Here's the drawing with two shaded views (mm, measured from the low corner). I have some questions. A direction names the side the tool comes from. Give positions to 0.01 mm unless a question says otherwise; leave off trailing zeros. Loops run counter-clockwise (first coordinate to the right, second up) from the corner with the lowest first, then second, coordinate; pieces in that order, holes last. Notation, with made-up numbers: M 32,77 L 48,77 A26 cw 48,91 Z; hole C 56.5,85.5 d9. An arc over 180 degrees is marked long. Put each result on its own line as item: value. Start each with the question number.
1) Imagine slicing it at B-B (z = 5.5). State how many separate pieces and enclosed holes the cut face has, then the cut area to 3 significant figures.
2) For the marked faces 4 and 5, which set-ups out of +Z, -Z, +X, -X, +Y, -Y let a thin tool reach every point of the face, with its end or its side?
3) Imagine slicing it at A-A (y = 5). Write out the boundary of the cut face in (x, z) (1 decimal).
4) If we mould it in two halves opening along X, with no side actions, what happens to the marked faces 1, 2 and 3? For each: +X half, -X half, draft (parallel to the pull), parting line (faces both ways), or undercut.
5) Please list where these lines run through material, in increasing order: line 1 along X through (y, z) = (1.5, 2.5); line 2 along X through (y, z) = (2.75, 5.25); line 3 along X through (y, z) = (4.5, 7) (1 decimal). Write a range as from..to.
6) For P1, Ø1.6, axis at y = 2, z = 3, coming from the -X side; P2, Ø1, axis at x = 41, z = 3.5, coming from the +Y side (1 decimal); P3, Ø3, axis at x = 46.5, z = 6, coming from the +Y side (1 decimal), each with a flat end and sliding along its axis, tell me the tip position at first contact or that it passes through.
7) Imagine slicing it at C-C (x = 4.5). Write out the boundary of the cut face in (y, z) (1 decimal).
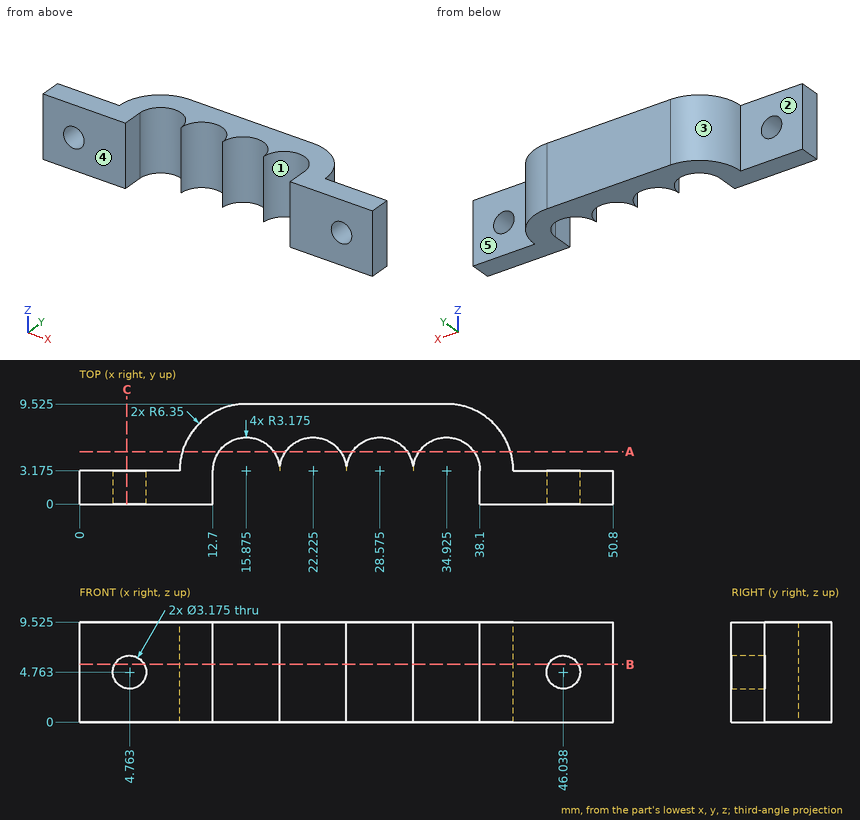
Recorded:
1. separate pieces: 3
1. enclosed holes: 0
1. area: 184 mm²
2. face 4: +Z, -Z, +X, -X, -Y
2. face 5: +Z, -Z, +X, +Y
3. outline: M 9.8,0 L 13.3,0 L 13.3,9.5 L 9.8,9.5 Z; M 18.5,0 L 19.6,0 L 19.6,9.5 L 18.5,9.5 Z; M 24.8,0 L 26,0 L 26,9.5 L 24.8,9.5 Z; M 31.2,0 L 32.3,0 L 32.3,9.5 L 31.2,9.5 Z; M 37.5,0 L 41,0 L 41,9.5 L 37.5,9.5 Z
4. face 1: undercut
4. face 2: draft
4. face 3: -X half
5. line 1: 0..12.7, 38.1..50.8
5. line 2: 0..3.25, 6.27..12.7, 38.1..44.53, 47.55..50.8
5. line 3: 9.7..13, 18.8..19.3, 25.1..25.7, 31.5..32, 37.8..41.1
6. P1: x = 0
6. P2: y = 6.2
6. P3: y = 3.2
7. outline: M 0,0 L 3.2,0 L 3.2,3.2 L 0,3.2 Z; M 0,6.3 L 3.2,6.3 L 3.2,9.5 L 0,9.5 Z
